Source: CAD feature listing. Evaluate the final solid. Frame: model axes, mm. A direction names the side the tool comes from. Give positions to 0.01 mm unless a question says otherwise; leave off trailing zeros. Order: outer loops, then holes, each group sorted by start corner. A loop starts at its lowest first (then second) coordinate and runs counter-clockwise, first axis right, second up. Notation, with made-up numbers: (80.5, -31.75) - (94.5, -31.75) arc R24 cw to (94.5, -0.75) - close; hole circle Ø2 at (71.25, 48). An arc over 180 degrees is marked (long way). Write each question's results on one line, items separated by ' | '. Start each with the question number.
Item 1: Section D-D on x = 8. Output: boundary loops of the cut face in (y, z).
Item 2: Mould query, pull axis X, two halves, no side actions, for faces 3 (the flat face through (16, 10, 6)), 4 (the flat face through (6, 4, 6)), 5 (the flat face through (26, 24, 6)). Classes: released by +X, released by -X, zero draft, split by the parting line, or undercut.
Item 3: Section B-B on y = 34. Output: boundary loops of the cut face in (x, z).
Item 4: Set-up query: faces 1 (the cylindrical face through (35.4, 3.43, 6.08)), 2 (the flat face through (14, 45, 6)). Return all of +Z, -Z, +X, -X, +Y, -Y with unobstructed straight access to the full face (end or side cutting, diameter ignored); none if empty.
Item 5: Line query: line 1 along X through (y, z) = (15, 6.5); line 2 along Z through (x, y) = (5, 0.9); line 3 along X through (y, z) = (45.5, 11.75). Output: solid intervals per line, ascending.
Item 6: Section A-A on y = 22. Output: boundary loops of the cut face in (x, z).
Item 7: Contact query for flat-ended pins moving along their axis: pin 1 Ø5.5 at (x, z) = (30.5, 4.5) entering from +Y; pin 2 Ø2.5 at (x, z) = (5, 7.52) entering from +Y; pin 3 Ø3.5 at (y, z) = (23.5, 5) entering from -X; pin 4 Ø3.5 at (y, z) = (22, 7.5) entering from +X. Output: stop coordinate, or through.
Item 8: Section C-C on x = 31. Output: boundary loops of the cut face in (y, z).
```python
from build123d import *

# Parameters (mm, degrees)
EXTRUDE_1_DEPTH          = 12
CUT_EXTRUDE_1_DEPTH      = 15
CUT_EXTRUDE_1_DEPTH_BACK = 15
SKETCH_2_R               = 1.45
SKETCH_3_R               = 1.45
CUT_EXTRUDE_2_DEPTH      = 15
FILLET_2_R               = 5
FILLET_3_R               = 2
CHAMFER_1_SIZE           = 2
SKETCH_4_W               = 12
SKETCH_4_H               = 8
EXTRUDE_2_DEPTH          = 10
CHAMFER_2_SIZE           = 5
CHAMFER_3_SIZE           = 1


with BuildPart() as part:
    # 草图1 → 凸台-拉伸1 (new body)
    with BuildSketch(Plane.XY):
        Polygon((0, 0), (13, 0), (13, 46), (23, 46), (23, 0), (36, 0), (36, 4), (26, 4), (26, 48), (10, 48), (10, 4), (0, 4), align=None)
    extrude(amount=EXTRUDE_1_DEPTH)

    # 草图2 → 切除-拉伸1 (cut, two sides: drawn at the far end of the back side and taken through both)
    with BuildSketch(Plane(origin=(13, 0, 0), x_dir=(0, 0, -1), z_dir=(1, 0, 0)).offset(-CUT_EXTRUDE_1_DEPTH_BACK)):
        with Locations(Location((-6, 34, 0), (0, 0, 180))):
            Circle(SKETCH_2_R)
    extrude(amount=CUT_EXTRUDE_1_DEPTH + CUT_EXTRUDE_1_DEPTH_BACK, mode=Mode.SUBTRACT)

    # 草图3 → 切除-拉伸2 (cut)
    with BuildSketch(Plane(origin=(0, 4, 0), x_dir=(1, 0, 0), z_dir=(0, 1, 0))):
        with Locations(Location((5, -7.519173445, 0), (0, 0, 180))):
            Circle(SKETCH_3_R)
        with Locations(Location((31, -7.519173445, 0), (0, 0, 180))):
            Circle(SKETCH_3_R)
    extrude(amount=-CUT_EXTRUDE_2_DEPTH, mode=Mode.SUBTRACT)

    # 圆角2
    fillet_2_edges = [part.edges().sort_by_distance(p)[0] for p in [
        (10, 48, 6),
        (26, 48, 6),
    ]]
    fillet(fillet_2_edges, radius=FILLET_2_R)

    # 圆角3
    fillet_3_edges = [part.edges().sort_by_distance(p)[0] for p in [
        (0, 4, 6),
        (36, 4, 6),
    ]]
    fillet(fillet_3_edges, radius=FILLET_3_R)

    # 倒角1
    chamfer_1_edges = [part.edges().sort_by_distance(p)[0] for p in [
        (23, 46, 6),
        (13, 46, 6),
    ]]
    chamfer(chamfer_1_edges, length=CHAMFER_1_SIZE)

    # 草图4 → 凸台-拉伸2 (add)
    with BuildSketch(Plane(origin=(13, 0, 0), x_dir=(0, 0, -1), z_dir=(1, 0, 0))):
        with Locations((-6, 4)):
            Rectangle(SKETCH_4_W, SKETCH_4_H)
    extrude(amount=EXTRUDE_2_DEPTH)

    # 倒角2
    chamfer_2_edges = [part.edges().sort_by_distance(p)[0] for p in [
        (13, 8, 6),
        (23, 8, 6),
    ]]
    chamfer(chamfer_2_edges, length=CHAMFER_2_SIZE - 0.0001)  # a hair under: the kernel refuses the full size

    # 倒角3
    chamfer_3_edges = [part.edges().sort_by_distance(p)[0] for p in [
        (10, 4, 6),
        (26, 4, 6),
    ]]
    chamfer(chamfer_3_edges, length=CHAMFER_3_SIZE)


solid = part.part
```
Evaluation:
1) outline: (0, 0) - (4, 0) - (4, 12) - (0, 12) - close
2) face 3: undercut | face 4: zero draft | face 5: released by +X
3) outline: (10, 0) - (13, 0) - (13, 4.55) - (10, 4.55) - close; (10, 7.45) - (13, 7.45) - (13, 12) - (10, 12) - close; (23, 0) - (26, 0) - (26, 4.55) - (23, 4.55) - close; (23, 7.45) - (26, 7.45) - (26, 12) - (23, 12) - close
4) face 1: +Z, -Z, +X, +Y | face 2: +Z, -Z
5) line 1: x = 10 to 13, 23 to 26 | line 2: z = 0 to 6.07, 8.97 to 12 | line 3: x = 10.67 to 14.5, 21.5 to 25.33
6) outline: (10, 0) - (13, 0) - (13, 12) - (10, 12) - close; (23, 0) - (26, 0) - (26, 12) - (23, 12) - close
7) pin 1: stops at y = 4 | pin 2: passes through | pin 3: stops at x = 10 | pin 4: stops at x = 26
8) outline: (0, 0) - (4, 0) - (4, 6.07) - (0, 6.07) - close; (0, 8.97) - (4, 8.97) - (4, 12) - (0, 12) - close
